Geometry check sheet. Reference: the model listing, model coordinates, mm. Round coordinates to 2 decimals unless told otherwise and drop trailing zeros. Write each loop counter-clockwise with the first axis right and the second up, starting at its lowest first coordinate (ties: lowest second). Pieces come first, ordered by that corner, then holes.
Item 1: Cross-section at A-A (z = 0). Enter the section's corners in (x, y), then the cut area to 3 significant figures.
Item 2: Scan lines: probe 1 along Y at (x, z) = (-42.05, 0); probe 2 along X at (y, z) = (1.25, -37.5); probe 3 along Z at (x, y) = (10, 3.5). Record each from-to range of solid material in increasing order.
Item 3: Draft check along Z on faces 1 (the face through (35.339, 3.451, 27.097)), 2 (the face through (0.59, 4.43, -42.77)), 3 (the face through (8.904, 3.451, 40.096)). Enter one of: pulls with the +Z half, pulls with the -Z half, needs draft (parallel to the pull), parting line crosses it, or undercut.
Item 4: Cross-section at D-D (x = 35). Enter the section's corners in (y, z), then the cut area to 3 significant figures.
Item 5: Depth check by flat-ended pin: P1, Ø2, axis at y = 4, z = 10, coming from the +X side; P2, Ø4, axis at y = 6, z = 16, coming from the -X side; P3, Ø1.5, axis at y = 2, z = 12.5, coming from the +X side. Enter the tip coordinate at first touch or a pass-through.
Item 6: Cross-section at B-B (x = 0). Enter the section's corners in (y, z).
Item 7: Cross-section at C-C (z = 32). Enter the section's corners in (x, y).
Autodesk Inventor part; units mm, degrees
ref_plane "YZ Plane" through (0, 0, 0) normal (1, 0, 0) x (0, 1, 0)
ref_plane "XZ Plane" through (0, 0, 0) normal (0, 1, 0) x (-1, 0, 0)
ref_plane "XY Plane" through (0, 0, 0) normal (0, 0, 1) x (1, 0, 0)
sketch "Sketch1" plane through (0, 0, 0) normal (0, 1, 0) x (-1, 0, 0)
  circle A0 centre (0, 0) radius 41.073
  circle A1 centre (0, 0) radius 44.5315
  dimension "d0" = 82.146
  dimension "d1" = 89.063
extrude "Extrusion1" add sketch "Sketch1" along normal blind 7
sketch "Sketch3" plane through (0, 0, 0) normal (0, 0, 1) x (1, 0, 0)
  circle A0 centre (0, 3.5) radius 1.1
  point P0 (0, 0)
  dimension "d4" = 2.2
extrude "Extrusion2" cut sketch "Sketch3" along normal blind 57 and the other way blind 58.5
sketch "Sketch4" plane through (0, 0, 0) normal (1, 0, 0) x (0, 1, 0)
  circle A0 centre (3.5, 0) radius 1.1
  point P0 (0, 0)
  dimension "d9" = 2.2
extrude "Extrusion3" cut sketch "Sketch4" along normal blind 57 and the other way blind 58.5
properties part number "Sensing Gripper Crown"
Resolved:
1. outline: (-44.53, 0) - (-41.07, 0) - (-41.07, 2.4) - (-44.53, 2.4) - close; (-44.53, 4.6) - (-41.07, 4.6) - (-41.07, 7) - (-44.53, 7) - close; (41.07, 0) - (44.53, 0) - (44.53, 2.4) - (41.07, 2.4) - close; (41.07, 4.6) - (44.53, 4.6) - (44.53, 7) - (41.07, 7) - close
1. area: 33.2 mm2
2. probe 1: y = 0 to 2.4, 4.6 to 7
2. probe 2: x = -24.02 to -16.76, 16.76 to 24.02
2. probe 3: z = -43.39 to -39.84, 39.84 to 43.39
3. face 1: parting line crosses it
3. face 2: needs draft
3. face 3: undercut
4. outline: (0, -27.53) - (7, -27.53) - (7, -21.49) - (0, -21.49) - close; (0, 21.49) - (7, 21.49) - (7, 27.53) - (0, 27.53) - close
4. area: 84.5 mm2
5. P1: stops at x = 43.61
5. P2: stops at x = -42.27
5. P3: stops at x = 42.95
6. outline: (0, -44.53) - (2.4, -44.53) - (2.4, -41.07) - (0, -41.07) - close; (0, 41.07) - (2.4, 41.07) - (2.4, 44.53) - (0, 44.53) - close; (4.6, -44.53) - (7, -44.53) - (7, -41.07) - (4.6, -41.07) - close; (4.6, 41.07) - (7, 41.07) - (7, 44.53) - (4.6, 44.53) - close
7. outline: (-30.97, 0) - (-25.75, 0) - (-25.75, 7) - (-30.97, 7) - close; (25.75, 0) - (30.97, 0) - (30.97, 7) - (25.75, 7) - close
